Here's how the part is built. I have some questions about the finished solid (model axes, mm). Face numbers are marked on the shaded views. Give positions to 0.01 mm unless a question says otherwise; leave off trailing zeros. Loops run counter-clockwise (first coordinate to the right, second up) from the corner with the lowest first, then second, coordinate; pieces in that order, holes last. Notation, with made-up numbers: (80, 56) - (130, 56) arc R25 ccw to (130, 81) - close; hole circle Ø8 at (-12.75, 32.25). An arc over 180 degrees is marked (long way). Return JSON: item names as keys, results as strings. Group by question number.
(1) I need wall thicknesses on probe 1 along Z at (x, y) = (1.25, -0.5); probe 2 along X at (y, z) = (-0.15, 0.5); probe 3 along X at (y, z) = (-0.5, 2). Which ranges of each line are inside material? Lowest first, please. Write a range as [from, to].
(2) If we section it at B-B (x = 0): Please give me the cut outline in (y, z).
(3) If we section it at D-D (z = -1): State how many separate pieces and enclosed holes the cut face has, then the cut area to 3 significant figures.
(4) If we section it at C-C (y = -0.1): Please give me the cut outline in (x, z), then the cut area to 3 significant figures.
(5) If we section it at A-A (z = 0): Please give me the cut outline in (x, y), then the cut area to 3 significant figures.
(6) If we mould it in two halves opening along Z, with no side actions, what happens to the marked faces 1, 2 and 3? For each: released by +Z, released by -Z, zero draft, split by the parting line, or undercut.
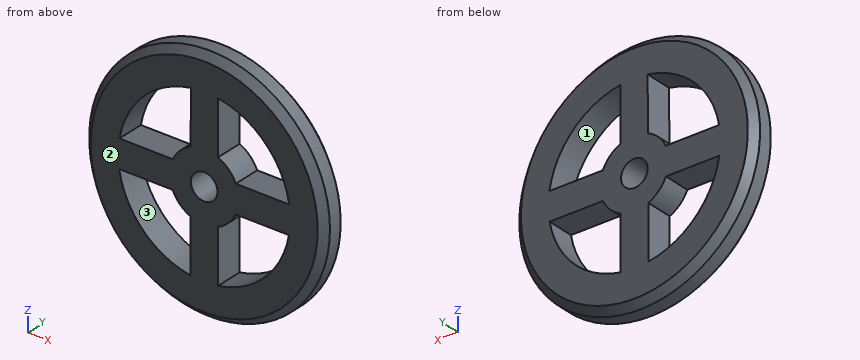
```python
from build123d import *

# Parameters (mm, degrees)
F0_R     = 3.5
F0_R_2   = 2.5
F1_DEPTH = 0.8
F2_SIZE  = 0.2
F4_DEPTH = 0.8
F6_R     = 0.386
F7_DEPTH = 25


with BuildPart() as f1:
    # F0 (on Front) → F1 (new body)
    with BuildSketch(Plane.XZ):
        Circle(F0_R)
        Circle(F0_R_2, mode=Mode.SUBTRACT)
    extrude(amount=F1_DEPTH)

    # F2
    f2_edges = [f1.edges().sort_by_distance(p)[0] for p in [
        (3.5, -0.4, 0),
        (-3.5, 0, 0),
        (-3.5, -0.8, 0),
    ]]
    chamfer(f2_edges, length=F2_SIZE)

    # F3 (on Front) → F4 (join)
    with BuildSketch(Plane.XZ):
        with BuildLine():
            Line((0.4040931107, -2.4671256064), (0.4040931107, -0.914717857))
            ThreePointArc((0.4040931107, -0.914717857), (0.7043653121, -0.7098376625), (0.9115631819, -0.411160024))
            Line((0.9115631819, -0.411160024), (2.463924442, -0.4231741297))
            ThreePointArc((2.463924442, -0.4231741297), (2.4909647835, -0.2123545325), (2.5, 0))
            ThreePointArc((2.5, 0), (2.4925336023, 0.1930705612), (2.4701790067, 0.3849878892))
            Line((2.4701790067, 0.3849878892), (0.9178177466, 0.3970019949))
            ThreePointArc((0.9178177466, 0.3970019949), (0.7098376625, 0.7043653121), (0.4040931107, 0.914717857))
            Line((0.4040931107, 0.914717857), (0.4040931107, 2.4671256064))
            ThreePointArc((0.4040931107, 2.4671256064), (0.0096738403, 2.4999812833), (-0.3849878892, 2.4701790067))
            Line((-0.3849878892, 2.4701790067), (-0.3970019949, 0.9178177466))
            ThreePointArc((-0.3970019949, 0.9178177466), (-0.7016132963, 0.7125579152), (-0.9115631819, 0.411160024))
            Line((-0.9115631819, 0.411160024), (-2.463924442, 0.4231741297))
            ThreePointArc((-2.463924442, 0.4231741297), (-2.4999251335, 0.0193475357), (-2.4701790067, -0.3849878892))
            Line((-2.4701790067, -0.3849878892), (-0.9178177466, -0.3970019949))
            ThreePointArc((-0.9178177466, -0.3970019949), (-0.7098376625, -0.7043653121), (-0.4040931107, -0.914717857))
            Line((-0.4040931107, -0.914717857), (-0.4040931107, -2.4671256064))
            ThreePointArc((-0.4040931107, -2.4671256064), (0, -2.5), (0.4040931107, -2.4671256064))
        make_face()
    extrude(amount=F4_DEPTH)

    # F6 (on face) → F7 (cut)
    with BuildSketch(Plane.XZ.offset(0.8)):
        Circle(F6_R)
    extrude(amount=-F7_DEPTH, mode=Mode.SUBTRACT)


solid = f1.part
```
Values:
{
 "1": {"probe 1": "[-3.27, -2.17], [-0.41, 0.39], [2.17, 3.27]", "probe 2": "[-3.41, -2.45], [-0.87, 0.87], [2.45, 3.41]", "probe 3": "[-2.87, -1.5], [-0.39, 0.4], [1.5, 2.87]"},
 "2": {"outline": "(-0.8, -3.3) - (-0.6, -3.5) - (-0.2, -3.5) - (0, -3.3) - (0, -0.39) - (-0.8, -0.39) - close; (-0.8, 0.39) - (0, 0.39) - (0, 3.3) - (-0.2, 3.5) - (-0.6, 3.5) - (-0.8, 3.3) - close"},
 "3": {"separate pieces": "3", "enclosed holes": "0", "area": "2.26 mm2"},
 "4": {"outline": "circle Ø6.8 at (0, 0); hole (-2.47, -0.38) arc R2.5 ccw to (-0.4, -2.47) - (-0.4, -0.91) arc R1 cw to (-0.92, -0.4) - close; hole (-2.46, 0.42) - (-0.91, 0.41) arc R1 cw to (-0.4, 0.92) - (-0.38, 2.47) arc R2.5 ccw to start; hole circle Ø0.77 at (0, 0); hole (0.4, -2.47) arc R2.5 ccw to (2.46, -0.42) - (0.91, -0.41) arc R1 cw to (0.4, -0.91) - close; hole (0.4, 0.91) arc R1 cw to (0.92, 0.4) - (2.47, 0.38) arc R2.5 ccw to (0.4, 2.47) - close", "area": "24.2 mm2"},
 "5": {"outline": "(-3.5, -0.6) - (-3.3, -0.8) - (-0.39, -0.8) - (-0.39, 0) - (-3.3, 0) - (-3.5, -0.2) - close; (0.39, -0.8) - (3.3, -0.8) - (3.5, -0.6) - (3.5, -0.2) - (3.3, 0) - (0.39, 0) - close", "area": "4.90 mm2"},
 "6": {"face 1": "undercut", "face 2": "zero draft", "face 3": "undercut"}
}
